For this review, use the dimensioned drawing (mm, ordinates from the lowest corner) and the shaded views. Coordinates: 2 decimals unless noted, no trailing zeros. Write each loop counter-clockwise with the first axis right and the second up, starting at its lowest first coordinate (ties: lowest second). Pieces come first, ordered by that corner, then holes. Notation, with made-up numbers: (21.5, 68) - (60.5, 68) arc R13 ccw to (60.5, 87) - close; hole circle Ø3 at (29, 0). An arc over 180 degrees is marked (long way). Put each result on its own line as item: value.
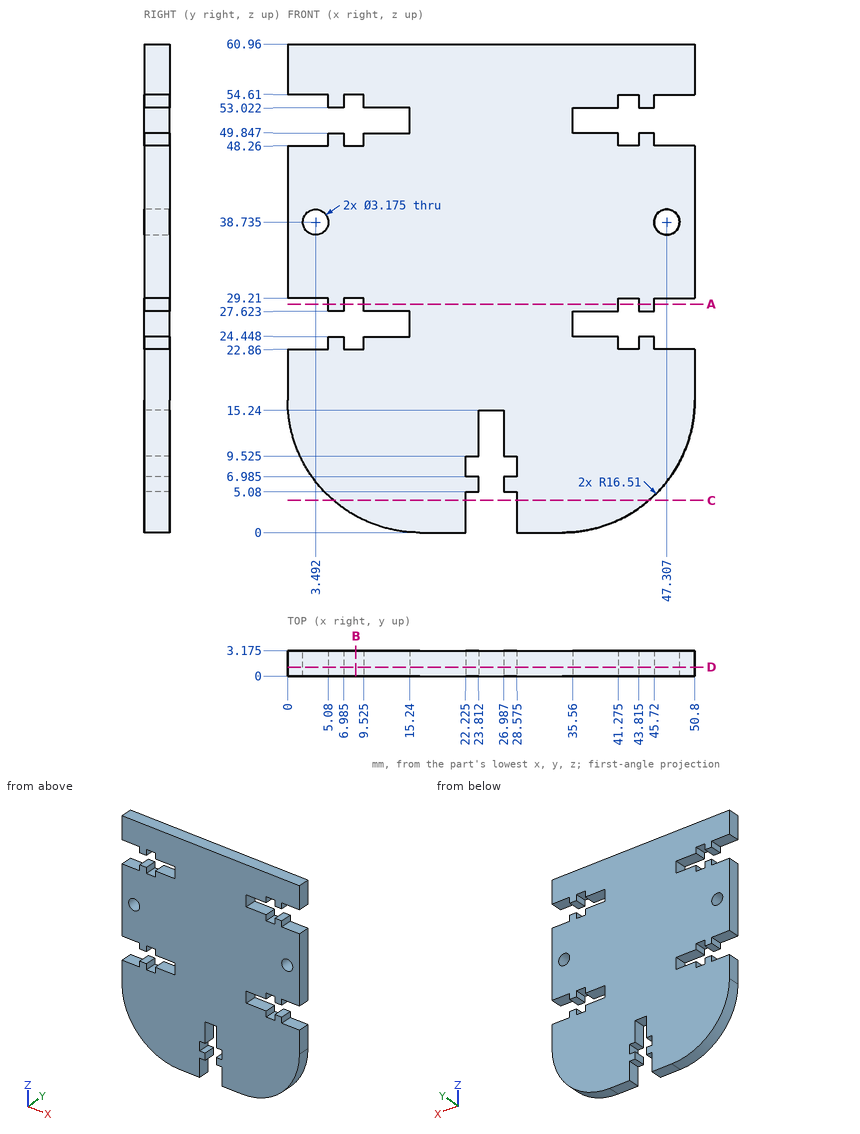
1. For pin 1 Ø0.8 at (y, z) = (1, 49) entering from -X; pin 2 Ø0.8 at (x, y) = (8.5, 2) entering from -Z; pin 3 Ø0.5 at (y, z) = (2, 53.5) entering from +X, all flat-tipped, find the tip position at first contact; note any pin that passes through.
Determined:
pin 1: stops at x = 5.08
pin 2: stops at z = 1.86
pin 3: stops at x = 45.72
2. Consider section B-B on x = 8.5. State the section outline as (y, z) points (1 decimal), plus the area to 3 significant figures.
Determined:
outline: (0, 2.1) - (3.2, 2.1) - (3.2, 22.9) - (0, 22.9) - close; (0, 29.2) - (3.2, 29.2) - (3.2, 48.3) - (0, 48.3) - close; (0, 54.6) - (3.2, 54.6) - (3.2, 61) - (0, 61) - close
area: 147 mm^2
3. Consider section D-D on y = 1.1. Give the number of separate pieces and of enclosed holes in the cut face, plus the area to 3 significant figures.
Determined:
separate pieces: 1
enclosed holes: 2
area: 2,600 mm^2
4. Consider section C-C on z = 4. State the section outline as (x, y) points (1 decimal).
Determined:
outline: (5.7, 0) - (22.2, 0) - (22.2, 3.2) - (5.7, 3.2) - close; (28.6, 0) - (45.1, 0) - (45.1, 3.2) - (28.6, 3.2) - close
5. To check wall thickness, follow probe 1 along X at (y, z) = (1.55, 48.5) (1 decimal); probe 2 along Z at (x, y) = (11, 1.15) (1 decimal); probe 3 along Z at (x, y) = (47.5, 2.7) (1 decimal). State the ranges of each line that lie inside material, in increasing order.
Determined:
probe 1: x = 5.1 to 7, 9.5 to 41.3, 43.8 to 45.7
probe 2: z = 0.9 to 24.4, 27.6 to 49.8, 53 to 61
probe 3: z = 6.6 to 22.9, 29.2 to 37.2, 40.3 to 48.3, 54.6 to 61
6. Consider section A-A on z = 28.5. State the section outline as (x, y) points (1 decimal), plus the area to 3 significant figures.
Determined:
outline: (5.1, 0) - (7, 0) - (7, 3.2) - (5.1, 3.2) - close; (9.5, 0) - (41.3, 0) - (41.3, 3.2) - (9.5, 3.2) - close; (43.8, 0) - (45.7, 0) - (45.7, 3.2) - (43.8, 3.2) - close
area: 113 mm^2
